```python
from build123d import *

# Parameters (mm, degrees)
F0_W     = 50.8
F0_H     = 50.8
F1_DEPTH = 25.4
F2_W     = 44.45
F2_H     = 44.45
F3_DEPTH = 19.05
F5_R     = 4.11241
F6_DEPTH = 19.1008
F4_R     = 1.5875
F7_DEPTH = 6.35


with BuildPart() as f1:
    # F0 (on Front) → F1 (new body)
    with BuildSketch(Plane.XZ):
        Rectangle(F0_W, F0_H)
    extrude(amount=F1_DEPTH)

    # F2 (on face) → F3 (cut)
    with BuildSketch(Plane.XZ.offset(25.4)):
        with Locations((3.175, -3.175)):
            Rectangle(F2_W, F2_H)
    extrude(amount=-F3_DEPTH, mode=Mode.SUBTRACT)

    # F5 (on face) → F6 (cut)
    with BuildSketch(Plane.XZ.offset(25.4)):
        with Locations((-19.05, 19.05)):
            Circle(F5_R)
    extrude(amount=-F6_DEPTH, mode=Mode.SUBTRACT)

    # F4 (on face) → F7 (cut)
    with BuildSketch(Plane.XZ.offset(6.35)):
        with Locations((19.05, -19.05)):
            Circle(F4_R)
    extrude(amount=-F7_DEPTH, mode=Mode.SUBTRACT)


solid = f1.part
```
Source: CAD feature listing. Evaluate the final solid. Frame: model axes, mm. A direction names the side the tool comes from. Give positions to 0.01 mm unless a question says otherwise; leave off trailing zeros. Write each loop counter-clockwise with the first axis right and the second up, starting at its lowest first coordinate (ties: lowest second). Pieces come first, ordered by that corner, then holes.
1. Section query A-A (x = 19.05). Return the cut outline in (y, z), then the cut area to 3 significant figures.
2. Section query B-B (z = -19.05). Return the cut outline in (x, y).
3. Access query for faces 5 (the face through (-19, -6.299, 19)), 6 (the face through (17.88, -3.219, -17.977)), 7 (the face through (-19.05, -16, -6)). Directions: +Z, -Z, +X, -X, +Y, -Y. A direction counts if a zero-diameter tool reaches every point of the face in a straight line with its end or side. Return the directions, or none.
4. Material intervals for line 1 along Z through (x, y) = (19.05, -1.5); line 2 along X through (y, z) = (-15.75, -2.5); line 3 along Z through (x, y) = (0, -12.75), sorted ascending.
5. Pull-direction query (Z, two-part tool) for faces 1 (the face through (3, -6.35, -3)), 2 (the face through (0, -13, 25.4)), 3 (the face through (-22.08, -15.98, 21.83)), 4 (the face through (5, -16, 19.05)); classes: +Z half, -Z half, draft (parallel to the pull), parting line (faces both ways), or undercut.
6. Section query D-D (x = 8.5). Return the cut outline in (y, z), then the cut area to 3 significant figures.
7. First-contact query: pin 1 (1 mm diameter, centred on x = -12.5, z = -18.5, fed in from -Y); pin 2 (10 mm diameter, centred on y = -13, z = 8, fed in from +X). Flat tips, straight axial feed; report the tip coordinate or a pass-through.
8. Section query C-C (y = -20.75). Return the cut outline in (x, z).
Output values:
1. outline: (-25.4, 19.05) - (-6.35, 19.05) - (-6.35, -17.46) - (0, -17.46) - (0, 25.4) - (-25.4, 25.4) - close; (-6.35, -25.4) - (0, -25.4) - (0, -20.64) - (-6.35, -20.64) - close
1. area: 423 mm2
2. outline: (-25.4, -25.4) - (-19.05, -25.4) - (-19.05, -6.35) - (17.46, -6.35) - (17.46, 0) - (-25.4, 0) - close; (20.64, -6.35) - (25.4, -6.35) - (25.4, 0) - (20.64, 0) - close
3. face 5: -Y
3. face 6: +Y, -Y
3. face 7: -Z, +X, -Y
4. line 1: z = -25.4 to -20.64, -17.46 to 25.4
4. line 2: x = -25.4 to -19.05
4. line 3: z = 19.05 to 25.4
5. face 1: draft
5. face 2: +Z half
5. face 3: undercut
5. face 4: -Z half
6. outline: (-25.4, 19.05) - (-6.35, 19.05) - (-6.35, -25.4) - (0, -25.4) - (0, 25.4) - (-25.4, 25.4) - close
6. area: 444 mm2
7. pin 1: stops at y = -6.35
7. pin 2: stops at x = -19.05
8. outline: (-25.4, -25.4) - (-19.05, -25.4) - (-19.05, 14.94) arc R4.11 cw (long way) to (-14.94, 19.05) - (25.4, 19.05) - (25.4, 25.4) - (-25.4, 25.4) - close
